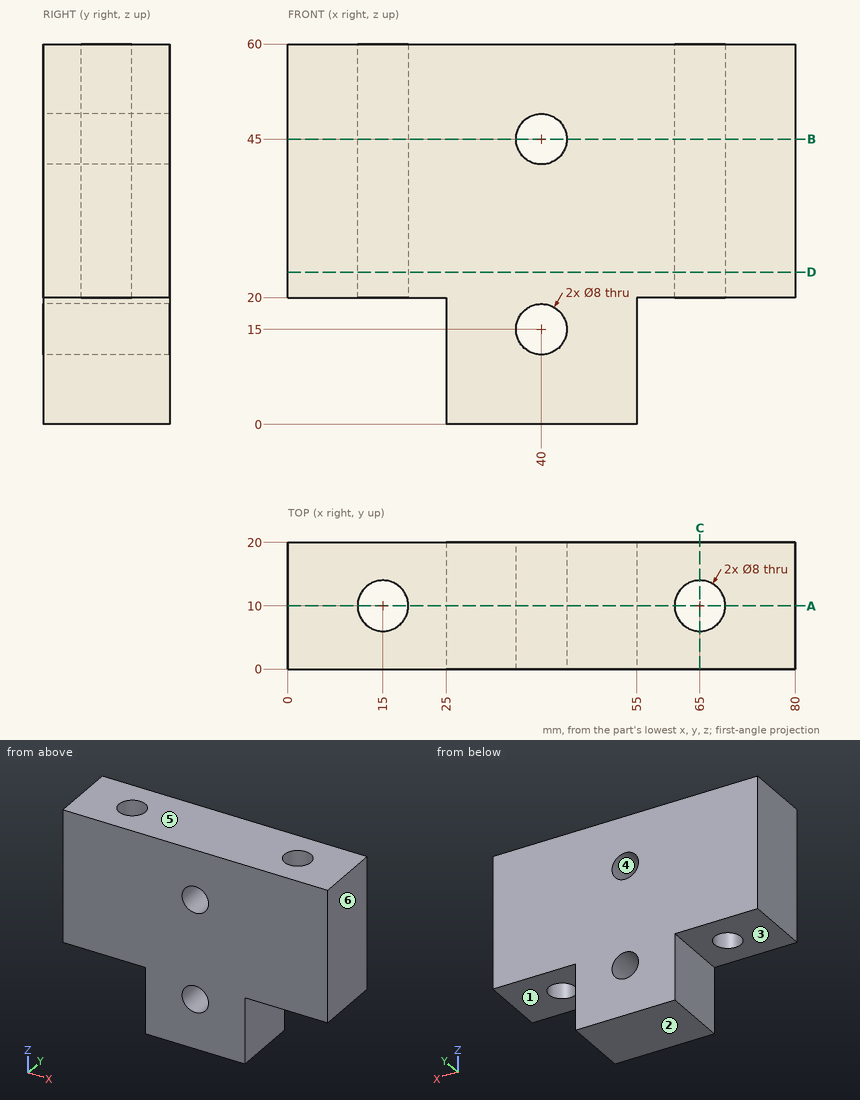
Design review of the part shown in the three views and the two pictorial views. Dimensions are in mm from the part's minimum x, y and z. A direction names the side the tool comes from. Round coordinates to 2 decimals unless told otherwise and drop trailing zeros. Order: outer loops, then holes, each group sorted by start corner. A loop starts at its lowest first (then second) coordinate and runs counter-clockwise, first axis right, second up. Notation, with made-up numbers: (25.25, 32.5) - (52.25, 32.5) arc R23 ccw to (52.25, 68.5) - close; hole circle Ø5 at (4, -21.75). An arc over 180 degrees is marked (long way). One line per question, with ' | ' between items.
Item 1: For P1, Ø4, axis at y = 4.5, z = 12.5, coming from the +X side; P2, Ø6, axis at x = 41, y = 14.5, coming from the -Z side; P3, Ø6, axis at x = 70, y = 11.5, coming from the -Z side; P4, Ø7, axis at x = 65, y = 10, coming from the -Z side, all flat-tipped, find the tip position at first contact; note any pin that passes through.
Checks:
P1: x = 55 | P2: z = 0 | P3: z = 20 | P4: through
Item 2: Wall thickness on line 1 (Z direction, x = 40, y = 4.5); line 2 (Y direction, x = 15, z = 49); line 3 (X direction, y = 4.25, z = 7.5): over which ranges is each line inside the solid? List them lowest first. Write a range as [from, to].
Checks:
line 1: [0, 11], [19, 41], [49, 60] | line 2: [0, 6], [14, 20] | line 3: [25, 55]
Item 3: Draft analysis for pull direction Z (two halves, no side actions). For the marked faces 4, 5 and 6, state which applies: +Z half, -Z half, draft (parallel to the pull), parting line (faces both ways), or undercut.
Checks:
face 4: undercut | face 5: +Z half | face 6: draft
Item 4: Take a section at A-A, the plane y = 10. Write out the cut boundary in (x, z), then the cut area to 3 significant figures.
Checks:
outline: (0, 20) - (11, 20) - (11, 60) - (0, 60) - close; (19, 20) - (25, 20) - (25, 0) - (55, 0) - (55, 20) - (61, 20) - (61, 60) - (19, 60) - close; (69, 20) - (80, 20) - (80, 60) - (69, 60) - close; hole circle Ø8 at (40, 15); hole circle Ø8 at (40, 45) | area: 3,060 mm²
Item 5: Machinability: for the marked faces 1, 2 and 3, which of the approach directions +Z, -Z, +X, -X, +Y, -Y give a long, thin tool a straight path to every point of the face, cutting with its end or side? Answer none if there is none.
Checks:
face 1: -Z, +X, +Y, -Y | face 2: -Z, +X, -X, +Y, -Y | face 3: -Z, -X, +Y, -Y
Item 6: Take a section at C-C, the plane x = 65. Write out the cut boundary in (y, z), then the cut area to 3 significant figures.
Checks:
outline: (0, 20) - (6, 20) - (6, 60) - (0, 60) - close; (14, 20) - (20, 20) - (20, 60) - (14, 60) - close | area: 480 mm²
Item 7: Take a section at B-B, the plane z = 45. Write out the cut boundary in (x, y).
Checks:
outline: (0, 0) - (36, 0) - (36, 20) - (0, 20) - close; (44, 0) - (80, 0) - (80, 20) - (44, 20) - close; hole circle Ø8 at (15, 10); hole circle Ø8 at (65, 10)
Item 8: Take a section at D-D, the plane z = 24. Write out the cut boundary in (x, y).
Checks:
outline: (0, 0) - (80, 0) - (80, 20) - (0, 20) - close; hole circle Ø8 at (15, 10); hole circle Ø8 at (65, 10)
